Autodesk Fusion 360 part; units mm, degrees
sketch "Boceto1" plane through (0, 0, 0) normal (0, 0, 1) x (1, 0, 0)
  circle A0 centre (0, 0) radius 19.5 construction
  line L0 (0, 0) -> (0, 18.75) construction
  line L1 (0, 18.75) -> (0.4305, 19.4952)
  line L2 (0, 18.75) -> (0.8606, 18.75) construction
  line L3 (0, 18.75) -> (-0.4305, 19.4952)
  line L4 (0, 18.75) -> (0.8606, 18.75) construction
  line L5 (-16.238, 9.375) -> (-17.0986, 9.3748)
  line L6 (-16.238, 9.375) -> (-16.6681, 10.1204)
  line L7 (-16.238, -9.375) -> (-16.6681, -10.1204)
  line L8 (-16.238, -9.375) -> (-17.0986, -9.3748)
  line L9 (0, -18.75) -> (0.4305, -19.4952)
  line L10 (0, -18.75) -> (-0.4305, -19.4952)
  line L11 (16.238, -9.375) -> (17.0986, -9.3748)
  line L12 (16.238, -9.375) -> (16.6681, -10.1204)
  line L13 (16.238, 9.375) -> (16.6681, 10.1204)
  line L14 (16.238, 9.375) -> (17.0986, 9.3748)
  circle A1 centre (0, 0) radius 19.5
  line L15 (0, 0) -> (0, -24.75) construction
  line L16 (0, 0) -> (0, -19.5) construction
  line L17 (0, 0) -> (19.5, 0) construction
  line L18 (0, -24.75) -> (-36.4194, -24.75) construction
  line L19 (-36.4194, -24.75) -> (0, -24.75) construction
  line L20 (30.7797, -24.75) -> (0, -24.75) construction
  line L21 (0, 0) -> (-19.5, 0) construction
  line L22 (-19.5, 0) -> (-19.5, -28.8)
  line L23 (0, 0) -> (19.396, 0) construction
  line L24 (19.396, 0) -> (19.396, -26.75) construction
  line L25 (19.396, -26.75) -> (21.396, -26.75) construction
  line L26 (19.396, -26.75) -> (17.396, -26.75) construction
  line L27 (13.9548, -13.6203) -> (13.9548, -24.75)
  arc A2 (13.926, -17.0313) -> (-19.4752, -10.2331) centre (0, 0) ccw
  line L28 (-19.5, -28.8) -> (-19.5, -30.8)
  line L29 (-19.5, -30.8) -> (28, -30.8)
  line L30 (13.9548, -24.75) -> (13.9548, -22.75)
  line L31 (13.9548, -22.75) -> (28, -22.75)
  line L32 (28, -22.75) -> (28, -30.8)
  line L33 (17.396, -26.75) -> (-6, -26.75) construction
  line L34 (0, 0) -> (0, -26.75) construction
  dimension "d1" = 39
  dimension "d2" = 18.75
  dimension "d3" = 59.988
  dimension "d4" = 0.8606
  dimension "d5" = 120.012
  dimension "d6" = 0.8606
  dimension "d8" = 360
  dimension "d9" = 39
  dimension "d10" = 24.75
  dimension "d13" = 19.5
  dimension "d14" = 28.8
  dimension "d15" = 19.396
  dimension "d16" = 26.75
  dimension "d17" = 2
  dimension "d18" = 2
  dimension "d19" = 11.1297
  dimension "d20" = 22
  dimension "d21" = 2
  dimension "d22" = 2
extrude "Extruir1" add sketch "Boceto1" along normal blind 44 contours L1 L3 A1 | A1 L22 L27 A2 | L13 L14 A1 | L5 L6 A1 | A1 L22 L27 L28 L29 L31 L32 | L11 L12 A1 | L7 L8 A1 | L9 L10 A1 makes body 1
sketch "Boceto2" plane through (0, -22.75, 0) normal (0, 1, 0) x (-1, 0, 0)
  line L0 (-28, 0) -> (-13.9548, 0)
  line L1 (-13.9548, 44) -> (-28, 44)
  line L2 (0, 0) -> (0, 21) construction
  line L3 (0, 21) -> (-19.396, 21) construction
  circle A0 centre (-19.396, 21) radius 2
  line L4 (-19.396, 21) -> (-19.396, 6) construction
  circle A1 centre (-19.396, 6) radius 2
  line L5 (-19.396, 6) -> (2.854, 6) construction
  line L6 (-19.396, 6) -> (-19.396, 0) construction
  line L7 (-19.396, 0) -> (5.604, 0) construction
  line L8 (-19.396, 6) -> (-19.396, 37.747) construction
  arc A2 (5.604, 0) -> (-29.313, 46.9893) centre (-109.7168, -49.2252) ccw
  line L9 (-109.7168, -49.2252) -> (5.604, 0) construction
  line L10 (-109.7168, -49.2252) -> (-29.313, 46.9893) construction
  line L11 (-29.313, 46.9893) -> (-29.313, 0)
  line L12 (-29.313, 0) -> (5.604, 0)
  dimension "d25" = 21
  dimension "d26" = 19.396
  dimension "d27" = 4
  dimension "d28" = 15
  dimension "d29" = 4
  dimension "d36" = 22.25
  dimension "d37" = 25
  dimension "d38" = 31.747
  dimension "d39" = 27
extrude "Extruir2" cut sketch "Boceto2" against normal blind 8.05 contours A0 | A1 bodies 1
ref_plane "PlanoDeObra1" through (0, -26.75, 0) normal (0, 1, 0) x (0, 0, 1)
sketch "Boceto3" plane through (0, -26.75, 0) normal (0, 1, 0) x (1, 0, 0)
  line L0 (0, 0) -> (19.792, 0) construction
  line L1 (19.792, 0) -> (-5.208, 0) construction
  dimension "d33" = 19.792
  dimension "d34" = 25
extrude "Extruir3" add sketch "Boceto2" against normal blind 4 separate body makes body 2
move_body "Desplazar1" bodies 2 to x (1, 0, 0) y (0, 1, 0) z (0, 0, 1) at (0, -2, 0)
combine "Combinar1" operation cut target body 1 tool bodies 2
Input: part model. Units: mm. Frame: model coordinates. A direction names the side the tool comes from. Round coordinates to 2 decimals unless told otherwise and drop trailing zeros. Loops run counter-clockwise (first coordinate to the right, second up) from the corner with the lowest first, then second, coordinate; pieces in that order, holes last. Notation, with made-up numbers: (3, 82.5) -> (22, 82.5) arc R14 ccw to (22, 92.5) -> close; hole circle Ø1 at (-23.5, 80). An arc over 180 degrees is marked (long way). One line per item, written item: value.
(1) Section C-C (x = -10.5). Return the cut outline in (y, z).
Geometry check:
outline: (-30.8, 0) -> (-16.43, 0) -> (-16.43, 44) -> (-30.8, 44) -> close; (16.43, 0) -> (19.33, 0) -> (19.33, 44) -> (16.43, 44) -> close
(2) Pin query (flat end, axial travel): pin 1 (22.5 mm diameter, centred on y = -18, z = 32, fed in from -X); pin 2 (7 mm diameter, centred on x = 19.5, z = 11, fed in from +Y); pin 3 (5 mm diameter, centred on x = 19.396, z = 6, fed in from +Y). Return the tip coordinate at first contact, or that it passes through.
Geometry check:
pin 1: x = -20.94
pin 2: y = 15.1
pin 3: y = 14.09
(3) Set-up query: faces 4 (the face through (15, -24.75, 17)), 5 (the face through (17.49, -29.76, 6.6)), 6 (the face through (13.955, -20, 22)), 7 (the face through (-19.5, -0.1, 21.7)), 8 (the face through (-19.5, -20, 22)). Return all of +Z, -Z, +X, -X, +Y, -Y with unobstructed straight access to the full face (end or side cutting, diameter ignored); none if empty.
Geometry check:
face 4: -Z, +X
face 5: -Y
face 6: +Z, -Z, +X
face 7: +Z, -Z
face 8: +Z, -Z, -X, -Y
(4) Mould query, pull axis X, two halves, no side actions, for faces 1 (the face through (3, -20, 44)), 2 (the face through (28, -30, 22)), 3 (the face through (9.631, 16.956, 21.692)). Classes: pulls with the +X half, pulls with the -X half, needs draft (parallel to the pull), parting line crosses it, or undercut.
Geometry check:
face 1: needs draft
face 2: pulls with the +X half
face 3: undercut
(5) Section D-D (z = 6). Give the number of separate pieces and of enclosed holes in the cut face, plus the area to 3 significant figures.
Geometry check:
separate pieces: 3
enclosed holes: 1
area: 684 mm2
(6) Material intervals for line 1 (Y direction, x = 6, z = 9.5); line 2 (Y direction, x = 15.5, z = 5); line 3 (Y direction, x = 14, z = 17), sorted ascending. Write a range as [from, to].
Geometry check:
line 1: [-30.8, -28.75], [-24.75, -18.55], [18.55, 21.17]
line 2: [-30.8, -28.75], [-24.75, -22.75], [-15.61, -11.83], [11.83, 15.61]
line 3: [-30.8, -28.75], [-24.75, -22.75], [-16.97, -13.57], [13.57, 16.97]
(7) Section A-A (y = -12). Return the cut outline in (x, z), plus the area to 3 significant figures.
Geometry check:
outline: (-19.5, 0) -> (-15.37, 0) -> (-15.37, 44) -> (-19.5, 44) -> close; (15.37, 0) -> (18.44, 0) -> (18.44, 44) -> (15.37, 44) -> close
area: 317 mm2
